from build123d import *

# Parameters (mm, degrees)
F1_DEPTH = 127
F2_W     = 119.324183
F2_H     = 39.356043
F2_W_2   = 118.48682
F2_H_2   = 11.723077
F2_H_3   = 23.446153
F2_W_3   = 122.88297
F2_W_4   = 21.771431
F2_H_4   = 60.29011
F2_W_5   = 28.889016
F2_W_6   = 53.172529
F2_H_5   = 59.871432
F3_DEPTH = 88.9
F5_DEPTH = 12.192


with BuildPart() as f1:
    # F0 (on Right) → F1 (new body, symmetric)
    with BuildSketch(Plane.YZ):
        with BuildLine():
            Line((-37.651766, -16.686577), (-37.651766, -58.902193))
            Line((-37.651766, -58.902193), (57.618611, -58.902193))
            Line((57.618611, -58.902193), (57.618611, 48.918769))
            Line((57.618611, 48.918769), (9.983422, 48.918769))
            ThreePointArc((9.983422, 48.918769), (-25.152108, 24.333902), (-37.651766, -16.686577))
        make_face()
    extrude(amount=F1_DEPTH, both=True)

    # F2 (on face) → F3 (cut)
    with BuildSketch(Plane.XY.offset(48.918769)):
        with Locations((-63.639564, 34.122527)):
            Rectangle(F2_W, F2_H)
        with Locations((-63.220882, -0.628023)):
            Rectangle(F2_W_2, F2_H_2)
        with Locations((-63.220882, -23.236814)):
            Rectangle(F2_W_2, F2_H_3)
        with Locations((61.441485, -23.236814)):
            Rectangle(F2_W_3, F2_H_3)
        with Locations((111.997254, 23.655494)):
            Rectangle(F2_W_4, F2_H_4)
        with Locations((79.549454, 23.655494)):
            Rectangle(F2_W_5, F2_H_4)
        with Locations((29.726374, 23.446155)):
            Rectangle(F2_W_6, F2_H_5)
    extrude(amount=-F3_DEPTH, mode=Mode.SUBTRACT)

    # F4 (on face) → F5 (join)
    with BuildSketch(Plane.XZ.offset(37.651766)):
        Polygon((-100.012504, -20.042138), (-107.780464, -20.042138), (-107.780464, -52.408643), (-100.012504, -52.408643), (-100.012504, -42.05136), (-90.626217, -52.408643), (-83.505586, -52.408643), (-100.012504, -32.988738), (-83.505586, -18.957859), (-88.360563, -16.686577), (-100.012504, -25.868108), align=None)
    extrude(amount=F5_DEPTH)


solid = f1.part
Verification items for the finished model (mm, model axes). A direction names the side the tool comes from. Round coordinates to 2 decimals unless told otherwise and drop trailing zeros. Write each loop counter-clockwise with the first axis right and the second up, starting at its lowest first coordinate (ties: lowest second). Pieces come first, ordered by that corner, then holes.
(1) Access from +Z, -Z, +X, -X, +Y, -Y to the whole of each face (thin tool, end or side, straight path). Record for faces 4 (the flat face through (-104, -44, -20.042)), 5 (the flat face through (-91.643, -43.662, -42.835)), 6 (the flat face through (29, 24, -39.981)).
Returned:
face 4: +Z, -X, -Y
face 5: +X, -Y
face 6: +Z
(2) Section check C-C (z = 20). Give the number of separate pieces and of enclosed holes in the cut face, plus the area to 3 significant figures.
Returned:
separate pieces: 1
enclosed holes: 5
area: 5,450 mm2
(3) Material ranges on line 1 (X direction, y = -16, z = -15.5); line 2 (X direction, y = 37.5, z = -11.5); line 3 (X direction, y = -2, z = -38.5), recorded low to high.
Returned:
line 1: x = -127 to -122.46, -3.98 to 0, 122.88 to 127
line 2: x = -127 to -123.3, -3.98 to 3.14, 56.31 to 65.1, 93.99 to 101.11, 122.88 to 127
line 3: x = -127 to -122.46, -3.98 to 3.14, 56.31 to 65.1, 93.99 to 101.11, 122.88 to 127
(4) Depth check by flat-ended pin: pin 1 Ø10 at (x, z) = (-74.5, -26.5) entering from -Y; pin 2 Ø6 at (x, y) = (3, -10.5) entering from +Z; pin 3 Ø3 at (x, z) = (76, 6.5) entering from -Y. Enter the tip coordinate at first touch or a pass-through.
Returned:
pin 1: stops at y = -37.65
pin 2: stops at z = 41.01
pin 3: stops at y = -11.51
(5) Mould release check, pull along Y, two halves, no side actions. Record for faces 1 (the flat face through (2, 57.619, -6)), 2 (the flat face through (-87, -44, -52.409)), 3 (the flat face through (-122.464, -23, -9)): pulls with the +Y half, pulls with the -Y half, needs draft (parallel to the pull), parting line crosses it, or undercut.
Returned:
face 1: pulls with the +Y half
face 2: needs draft
face 3: undercut
(6) Section check A-A (y = 40.5). Enter the section's corners in (x, z).
Returned:
outline: (-127, -58.9) - (127, -58.9) - (127, 48.92) - (122.88, 48.92) - (122.88, -39.98) - (101.11, -39.98) - (101.11, 48.92) - (93.99, 48.92) - (93.99, -39.98) - (65.1, -39.98) - (65.1, 48.92) - (56.31, 48.92) - (56.31, -39.98) - (3.14, -39.98) - (3.14, 48.92) - (-3.98, 48.92) - (-3.98, -39.98) - (-123.3, -39.98) - (-123.3, 48.92) - (-127, 48.92) - close
(7) Section check B-B (x = 31). Enter the section's corners in (y, z).
Returned:
outline: (-37.65, -58.9) - (57.62, -58.9) - (57.62, 48.92) - (53.38, 48.92) - (53.38, -39.98) - (-6.49, -39.98) - (-6.49, 41.65) arc R65.74 ccw to (-11.51, 38.22) - (-11.51, -39.98) - (-34.96, -39.98) - (-34.96, 4.48) arc R65.74 ccw to (-37.65, -16.69) - close
